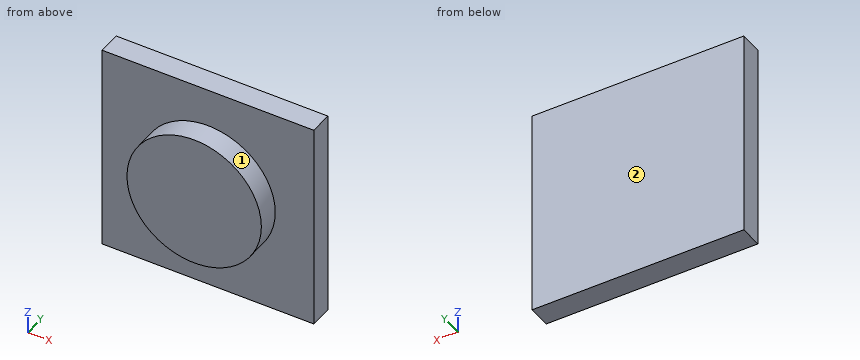
from build123d import *

# Parameters (mm, degrees)
F0_W     = 37
F0_H     = 37
F1_DEPTH = 4
F2_R     = 11.75
F3_DEPTH = 8


with BuildPart() as f1:
    # F0 (on Front) → F1 (new body)
    with BuildSketch(Plane.XZ):
        Rectangle(F0_W, F0_H)
    extrude(amount=F1_DEPTH)

    # F2 (on Front) → F3 (join)
    with BuildSketch(Plane.XZ):
        Circle(F2_R)
    extrude(amount=F3_DEPTH)


solid = f1.part
Design review of the part built by this model. Coordinates are the model's own, in mm. Face numbers are marked on the shaded views. A direction names the side the tool comes from. Coordinates: 2 decimals unless noted, no trailing zeros. Write each loop counter-clockwise with the first axis right and the second up, starting at its lowest first coordinate (ties: lowest second). Pieces come first, ordered by that corner, then holes. Notation, with made-up numbers: (-21.75, -25.75) - (-0.75, -25.75) arc R23 ccw to (-0.75, 4.25) - close; hole circle Ø10 at (-21.75, 73). An arc over 180 degrees is marked (long way). Use one line per item in the form item = value.
Q1. Machinability: for the marked faces 1 and 2, which of the approach directions +Z, -Z, +X, -X, +Y, -Y give a long, thin tool a straight path to every point of the face, cutting with its end or side? Answer none if there is none.
Taken from the geometry:
face_1 = -Y
face_2 = +Z, -Z, +X, -X, +Y
Q2. Consider section D-D (z = 12.5). Write out the cut boundary in (x, y).
Taken from the geometry:
outline = (-18.5, -4) - (18.5, -4) - (18.5, 0) - (-18.5, 0) - close
Q3. For probe 1 along Y at (x, z) = (13.5, -1); probe 2 along Z at (x, y) = (8.5, -4.25); probe 3 along Z at (x, y) = (-9, -6.5), list the stretches that pass through material, from the lowest coordinate up.
Taken from the geometry:
probe_1 = -4 to 0
probe_2 = -8.11 to 8.11
probe_3 = -7.55 to 7.55
Q4. Consider section B-B (x = 0). Write out the cut boundary in (y, z), plus the area to 3 significant figures.
Taken from the geometry:
outline = (-8, -11.75) - (-4, -11.75) - (-4, -18.5) - (0, -18.5) - (0, 18.5) - (-4, 18.5) - (-4, 11.75) - (-8, 11.75) - close
area = 242 mm^2
Q5. Consider section A-A (z = 0). Write out the cut boundary in (x, y), plus the area to 3 significant figures.
Taken from the geometry:
outline = (-18.5, -4) - (-11.75, -4) - (-11.75, -8) - (11.75, -8) - (11.75, -4) - (18.5, -4) - (18.5, 0) - (-18.5, 0) - close
area = 242 mm^2
Q6. Consider section C-C (x = -13). Write out the cut boundary in (y, z), plus the area to 3 significant figures.
Taken from the geometry:
outline = (-4, -18.5) - (0, -18.5) - (0, 18.5) - (-4, 18.5) - close
area = 148 mm^2
Q7. Insertion check: pin 1 Ø2 at (y, z) = (-6, 9) entering from -X. The pin has a flat end and moves straight along its axis. Give the tip position at first contact, or say it passes through.
Taken from the geometry:
pin_1 = -8.61
